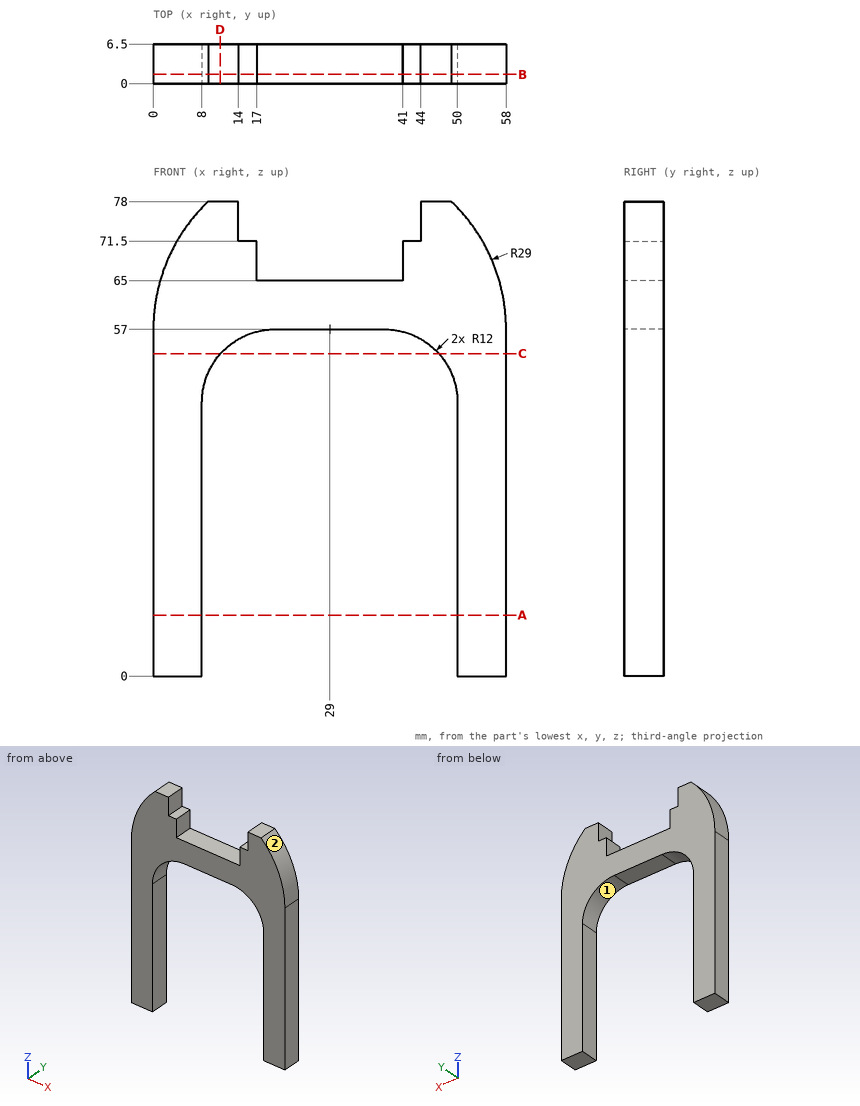
Geometry: see drawing. Coordinates: mm, zero at the bounding-box minimum. A direction names the side the tool comes from. Coordinates: 2 decimals unless noted, no trailing zeros. Order: outer loops, then holes, each group sorted by start corner. A loop starts at its lowest first (then second) coordinate and runs counter-clockwise, first axis right, second up. Notation, with made-up numbers: (24.5, -18.5) - (52.5, -18.5) arc R10 cw to (52.5, -0.5) - close; hole circle Ø7 at (47, -35). An arc over 180 degrees is marked (long way). Use one line per item in the form item = value.
1) Section D-D (x = 11). Return loops of the section in (y, z), then the cut area to 3 significant figures.
Solutions:
outline = (0, 52.94) - (6.5, 52.94) - (6.5, 78) - (0, 78) - close
area = 163 mm^2
2) Section A-A (z = 10). Return loops of the section in (x, y).
Solutions:
outline = (0, 0) - (8, 0) - (8, 6.5) - (0, 6.5) - close; (50, 0) - (58, 0) - (58, 6.5) - (50, 6.5) - close
3) Pin query (flat end, axial travel): pin 1 (3 mm diameter, centred on x = 20.5, y = 4.5, fed in from +Z); pin 2 (2 mm diameter, centred on y = 2.5, z = 73.5, fed in from -X); pin 3 (0.9 mm diameter, centred on x = 43, y = 3.5, fed in from +Z). Return the tip coordinate at first contact, or that it passes through.
Solutions:
pin_1 = 65
pin_2 = 4.49
pin_3 = 71.5
4) Set-up query: the marked faces 1 and 2. Return all of +Z, -Z, +X, -X, +Y, -Y with unobstructed straight access to the full face (end or side cutting, diameter ignored); none if empty.
Solutions:
face_1 = -Z, +Y, -Y
face_2 = +Z, +X, +Y, -Y
5) Section C-C (z = 53). Return loops of the section in (x, y), then the cut area to 3 significant figures.
Solutions:
outline = (0, 0) - (11.06, 0) - (11.06, 6.5) - (0, 6.5) - close; (46.94, 0) - (58, 0) - (58, 6.5) - (46.94, 6.5) - close
area = 144 mm^2
6) Section B-B (y = 1.5). Return loops of the section in (x, z), then the cut area to 3 significant figures.
Solutions:
outline = (0, 0) - (8, 0) - (8, 45) arc R12 cw to (20, 57) - (38, 57) arc R12 cw to (50, 45) - (50, 0) - (58, 0) - (58, 57) arc R29 ccw to (49, 78) - (44, 78) - (44, 71.5) - (41, 71.5) - (41, 65) - (17, 65) - (17, 71.5) - (14, 71.5) - (14, 78) - (9, 78) arc R29 ccw to (0, 57) - close
area = 1,720 mm^2
7) Ray query, L1, parallel to X at y = 6, z = 10; L2, parallel to Z at x = 35.5, y = 2.5; L3, parallel to X at y = 1.5, z = 46.5. Return the intervals inside material, ascending.
Solutions:
L1 = 0 to 8, 50 to 58
L2 = 57 to 65
L3 = 0 to 8.09, 49.91 to 58
